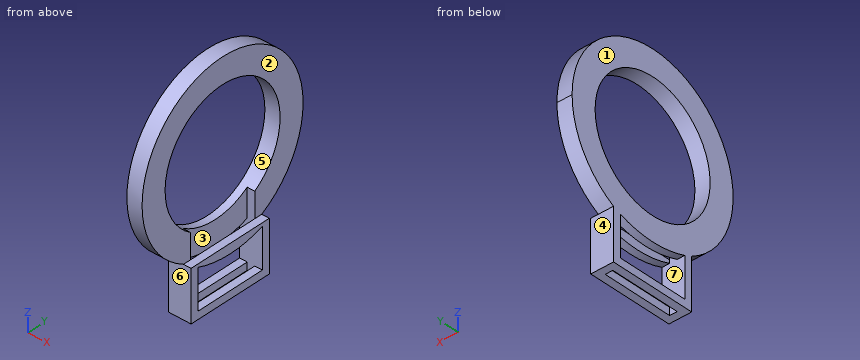
```python
from build123d import *

# Parameters (mm, degrees)
F1_DEPTH = 11.43
F0_R     = 31.75
F4_DEPTH = 7.62
F2_W     = 3.81
F2_H     = 35.56
F5_DEPTH = 76.2
F6_DEPTH = 76.2


with BuildPart() as f1:
    # F0 (on Right) → F1 (new body)
    with BuildSketch(Plane.YZ):
        with BuildLine():
            Line((-21.237904, -275.042741), (-64.417904, -275.042741))
            ThreePointArc((-64.417904, -275.042741), (-42.827904, -280.638212), (-21.237904, -275.042741))
        make_face()
        with BuildLine():
            ThreePointArc((-21.237904, -275.042741), (-42.827904, -280.638212), (-64.417904, -275.042741))
            Line((-64.417904, -275.042741), (-64.417904, -300.442741))
            Line((-64.417904, -300.442741), (-21.237904, -300.442741))
            Line((-21.237904, -300.442741), (-21.237904, -275.042741))
        make_face()
    extrude(amount=F1_DEPTH)

    # F0 (on Right) → F4 (join)
    with BuildSketch(Plane.YZ):
        with BuildLine():
            ThreePointArc((-21.237904, -275.042741), (-4.516822, -258.728476), (1.622096, -236.188212))
            ThreePointArc((1.622096, -236.188212), (-65.368168, -197.87713), (-64.417904, -275.042741))
            Line((-64.417904, -275.042741), (-21.237904, -275.042741))
        make_face()
        with Locations((-42.827904, -236.188212)):
            Circle(F0_R, mode=Mode.SUBTRACT)
    extrude(amount=F4_DEPTH)

    # F2 (on face) → F5 (cut)
    with BuildSketch(Plane(origin=(0, 0, -300.442741), x_dir=(1, 0, 0), z_dir=(0, 0, -1))):
        with Locations((5.715, 42.827904)):
            Rectangle(F2_W, F2_H)
    extrude(amount=-F5_DEPTH, mode=Mode.SUBTRACT)

    # F3 (on face) → F6 (cut)
    with BuildSketch(Plane.YZ.offset(11.43)):
        with BuildLine():
            Line((-60.607904, -276.645803), (-60.607904, -296.632741))
            Line((-60.607904, -296.632741), (-25.047904, -296.632741))
            Line((-25.047904, -296.632741), (-25.047904, -276.645803))
            ThreePointArc((-25.047904, -276.645803), (-42.827904, -279.858919), (-60.607904, -276.645803))
        make_face()
    extrude(amount=-F6_DEPTH, mode=Mode.SUBTRACT)


solid = f1.part
```
Can you work these out from the model? Positions are in its coordinate system, mm. Face numbers are marked on the shaded views. A direction names the side the tool comes from. Coordinates: 2 decimals unless noted, no trailing zeros. Loops run counter-clockwise (first coordinate to the right, second up) from the corner with the lowest first, then second, coordinate; pieces in that order, holes last.
Item 1: Suppose I cut it at D-D (z = -246.5). Please give me the cut outline in (x, y).
Answers below:
outline: (0, -86.07) - (7.62, -86.07) - (7.62, -72.86) - (0, -72.86) - close; (0, -12.8) - (7.62, -12.8) - (7.62, 0.41) - (0, 0.41) - close
Item 2: I'm going to push flat-ended pins straight in: pin 1 (3.5 mm diameter, centred on x = 3, z = -293.5, fed in from -Y); pin 2 (6 mm diameter, centred on y = -44.5, z = -205, fed in from -X); pin 3 (8 mm diameter, centred on y = -70, z = -240.5, fed in from +X) (3 decimals); pin 4 (2 mm diameter, centred on x = 4, y = -39, fed in from +Z). Where does each tip first touch, or does it pass through?
Answers below:
pin 1: stops at y = -64.42
pin 2: stops at x = 0
pin 3: passes through
pin 4: stops at z = -191.83
Item 3: Suppose I cut it at A-A (x = 2.5). Please give me the cut outline in (y, z).
Answers below:
outline: (-64.42, -300.44) - (-21.24, -300.44) - (-21.24, -275.04) arc R44.45 ccw (long way) to (-64.42, -275.04) - close; hole circle Ø63.5 at (-42.83, -236.19); hole (-60.61, -296.63) - (-25.05, -296.63) - (-25.05, -276.65) arc R50.8 cw to (-60.61, -276.65) - close
Item 4: Which directions (+Z, -Z, +X, -X, +Y, -Y) give clear straight access to the entire face, cutting with the end or side of a thin tool? Please do the marked faces 1, 2, 3, 4 and 5.
Answers below:
face 1: +Z, -Z, -X, +Y, -Y
face 2: +Z, +X, +Y, -Y
face 3: -Z
face 4: -Z, +X, -X, +Y
face 5: +X, -X
Item 5: If we mould it in two halves opening along Z, with no side actions, what happens to the marked faces 6 and 7? For each: released by +Z, released by -Z, zero draft, split by the parting line, or undercut.
Answers below:
face 6: zero draft
face 7: undercut
Item 6: Suppose I cut it at C-C (y = -30.5). Please give me the cut outline in (x, z), then the cut area to 3 significant figures.
Answers below:
outline: (0, -300.44) - (3.81, -300.44) - (3.81, -296.63) - (0, -296.63) - close; (0, -278.34) - (3.81, -278.34) - (3.81, -265.45) - (0, -265.45) - close; (0, -206.93) - (7.62, -206.93) - (7.62, -193.48) - (0, -193.48) - close; (7.62, -300.44) - (11.43, -300.44) - (11.43, -296.63) - (7.62, -296.63) - close; (7.62, -278.34) - (11.43, -278.34) - (11.43, -275.04) - (7.62, -275.04) - close
area: 193 mm2
Item 7: Suppose I cut it at B-B (y = -68.5). Please give me the cut outline in (x, z).
Answers below:
outline: (0, -272.48) - (7.62, -272.48) - (7.62, -254.87) - (0, -254.87) - close; (0, -217.51) - (7.62, -217.51) - (7.62, -199.9) - (0, -199.9) - close
Item 8: Please list where these lines run through material, in increasing order: L1, parallel to Y at x = 3, z = -290; L2, parallel to Z at x = 3.25, y = -40.5; L3, parallel to X at y = -36.5, z = -275.5.
Answers below:
L1: y = -64.42 to -60.61, -25.05 to -21.24
L2: z = -300.44 to -296.63, -279.81 to -267.85, -204.52 to -191.8
L3: x = 0 to 3.81, 7.62 to 11.43
